```python
from build123d import *

# Parameters (mm, degrees)
SKETCH1_R           = 20.5
SKETCH1_R_2         = 1.5875
SKETCH1_R_3         = 13.5
EXTRUDE1_DEPTH      = 1.5
BOSS_EXTRUDE1_START = -21.9577
SKETCH2_R           = 22
SKETCH2_R_2         = 20.5
BOSS_EXTRUDE1_DEPTH = 21.9577


with BuildPart() as part:
    # Sketch1 → Extrude1 (new body)
    # profile 1 of 4: a face of its own
    with BuildSketch(Plane.XY):
        Circle(SKETCH1_R)
        with Locations((-14.289419162, 8.25)):
            Circle(SKETCH1_R_2, mode=Mode.SUBTRACT)
        with Locations((0, -16.5)):
            Circle(SKETCH1_R_2, mode=Mode.SUBTRACT)
        with Locations((14.289419162, 8.25)):
            Circle(SKETCH1_R_2, mode=Mode.SUBTRACT)
        with Locations((-14.289419162, -8.25)):
            Circle(SKETCH1_R_2, mode=Mode.SUBTRACT)
        with Locations((14.289419162, -8.25)):
            Circle(SKETCH1_R_2, mode=Mode.SUBTRACT)
        with Locations((0, 16.5)):
            Circle(SKETCH1_R_2, mode=Mode.SUBTRACT)
        Circle(SKETCH1_R_3, mode=Mode.SUBTRACT)
    # profile 2 of 4: a face of its own
    with BuildSketch(Plane.XY):
        with Locations((-14.289419162, 8.25)):
            Circle(SKETCH1_R_2)
    # profile 3 of 4: a face of its own
    with BuildSketch(Plane.XY):
        with Locations((14.289419162, 8.25)):
            Circle(SKETCH1_R_2)
    # profile 4 of 4: a face of its own
    with BuildSketch(Plane.XY):
        with Locations((0, -16.5)):
            Circle(SKETCH1_R_2)
    extrude(amount=EXTRUDE1_DEPTH)

    # Sketch2 → Boss-Extrude1 (add)
    with BuildSketch(Plane.XY.offset(1.5).offset(BOSS_EXTRUDE1_START)):
        Circle(SKETCH2_R)
        Circle(SKETCH2_R_2, mode=Mode.SUBTRACT)
    extrude(amount=BOSS_EXTRUDE1_DEPTH)


solid = part.part
```
Geometry: final body of the model. Coordinates: model frame, mm. A direction names the side the tool comes from. Round coordinates to 2 decimals unless told otherwise and drop trailing zeros. Loops run counter-clockwise (first coordinate to the right, second up) from the corner with the lowest first, then second, coordinate; pieces in that order, holes last.
Item 1: Reachability of faces 4 (the flat face through (9.5, 10.1, 1.5)), 5 (the flat face through (13.4, -4.3, 0)) from +Z, -Z, +X, -X, +Y, -Y: full face, straight path, thin tool, end or side. Return the list, or none.
Checked values:
face 4: +Z, +X, -X, +Y, -Y
face 5: -Z
Item 2: Mould query, pull axis Y, two halves, no side actions, for faces 1 (the cylindrical face through (-4.769, -21.477, -9.633)), 2 (the flat face through (15, -15, -20.458)), 3 (the cylindrical face through (-0.34, 14.95, 0.74)). Classes: released by +Y, released by -Y, zero draft, split by the parting line, or undercut.
Checked values:
face 1: split by the parting line
face 2: zero draft
face 3: undercut
Item 3: Contact query for flat-ended pins moving along their axis: P1, Ø5, axis at x = -16, z = -1.5, coming from the +Y side; P2, Ø4, axis at x = -14.29, y = -8.25, coming from the -Z side; P3, Ø1, axis at x = -1.5, z = -17.5, coming from the +Y side. Output: stop coordinate, or through.
Checked values:
P1: stops at y = 17.37
P2: stops at z = 0
P3: stops at y = 21.98
Item 4: Section B-B, the plane y = 0. Output: boundary loops of the cut face in (x, z).
Checked values:
outline: (-22, -20.46) - (-20.5, -20.46) - (-20.5, 0) - (-13.5, 0) - (-13.5, 1.5) - (-22, 1.5) - close; (13.5, 0) - (20.5, 0) - (20.5, -20.46) - (22, -20.46) - (22, 1.5) - (13.5, 1.5) - close
Item 5: Section C-C, the plane y = -8.25. Output: boundary loops of the cut face in (x, z).
Checked values:
outline: (-20.39, -20.46) - (-18.77, -20.46) - (-18.77, 0) - (-15.88, 0) - (-15.88, 1.5) - (-20.39, 1.5) - close; (-12.7, 0) - (-10.69, 0) - (-10.69, 1.5) - (-12.7, 1.5) - close; (10.69, 0) - (12.7, 0) - (12.7, 1.5) - (10.69, 1.5) - close; (15.88, 0) - (18.77, 0) - (18.77, -20.46) - (20.39, -20.46) - (20.39, 1.5) - (15.88, 1.5) - close
Item 6: Section A-A, the plane x = 0. Output: boundary loops of the cut face in (y, z), plus the area to 3 significant figures.
Checked values:
outline: (-22, -20.46) - (-20.5, -20.46) - (-20.5, 0) - (-13.5, 0) - (-13.5, 1.5) - (-22, 1.5) - close; (13.5, 0) - (14.91, 0) - (14.91, 1.5) - (13.5, 1.5) - close; (18.09, 0) - (20.5, 0) - (20.5, -20.46) - (22, -20.46) - (22, 1.5) - (18.09, 1.5) - close
area: 82.1 mm2
Item 7: Line query: L1, parallel to Y at x = 0, z = 1.1; L2, parallel to Y at x = 0, z = -6.5; L3, parallel to Z at x = 5, y = -19.5. Output: solid intervals per line, ascending.
Checked values:
L1: y = -22 to -13.5, 13.5 to 14.91, 18.09 to 22
L2: y = -22 to -20.5, 20.5 to 22
L3: z = 0 to 1.5
Item 8: Section D-D, the plane x = 9. Output: boundary loops of the cut face in (y, z).
Checked values:
outline: (-20.07, -20.46) - (-18.42, -20.46) - (-18.42, 0) - (-10.06, 0) - (-10.06, 1.5) - (-20.07, 1.5) - close; (10.06, 0) - (18.42, 0) - (18.42, -20.46) - (20.07, -20.46) - (20.07, 1.5) - (10.06, 1.5) - close
